Verification items for the finished model (mm, model axes). A direction names the side the tool comes from. Coordinates: 2 decimals unless noted, no trailing zeros. Write each loop counter-clockwise with the first axis right and the second up, starting at its lowest first coordinate (ties: lowest second). Pieces come first, ordered by that corner, then holes. Notation, with made-up numbers: M 47,-17 L 70,-17 A22 ccw 70,12 Z; hole C 84,26 d11. An arc over 180 degrees is marked long. Answer in a Markdown table with one row per item.
from build123d import *

# Parameters (mm, degrees)
CROQUIS1_W               = 12.68
CROQUIS1_H               = 12.6
SALIENTE_EXTRUIR1_DEPTH  = 5
SALIENTE_EXTRUIR3_DEPTH  = 5
SALIENTE_EXTRUIR4_DEPTH  = 12.5
CROQUIS2_W               = 12.6
CROQUIS2_H               = 5
CORTAR_EXTRUIR1_DEPTH    = 127.5
CROQUIS3_W               = 4.8
CROQUIS3_H               = 5
CORTAR_EXTRUIR2_DEPTH    = 255
CROQUIS4_W               = 116.76
CROQUIS4_H               = 10
CROQUIS4_H_2             = 12.5
SALIENTE_EXTRUIR5_DEPTH  = 25
CROQUIS5_R               = 4.5
CORTAR_EXTRUIR3_DEPTH    = 155
CROQUIS6_R               = 7.7
CORTAR_EXTRUIR4_DEPTH    = 20.3
CROQUIS7_R               = 7.7
SALIENTE_EXTRUIR6_DEPTH  = 5
CORTAR_EXTRUIR5_DEPTH    = 25.2
CROQUIS9_W               = 1
CROQUIS9_H               = 10
CORTAR_EXTRUIR6_DEPTH    = 4.8
CROQUIS10_W              = 117.76
CROQUIS10_H              = 0.4
CORTAR_EXTRUIR7_DEPTH    = 10
CROQUIS11_R              = 2
CORTAR_EXTRUIR8_DEPTH    = 10
CROQUIS12_W              = 3
CROQUIS12_H              = 7.5
CORTAR_EXTRUIR9_DEPTH    = 220
CORTAR_EXTRUIR10_DEPTH   = 220
SALIENTE_EXTRUIR7_DEPTH  = 16.68
CROQUIS15_R              = 7.7
SALIENTE_EXTRUIR8_DEPTH  = 1
CROQUIS16_R              = 7.7
CROQUIS16_R_2            = 4.5
SALIENTE_EXTRUIR9_DEPTH  = 1.8
SALIENTE_EXTRUIR10_DEPTH = 1
CROQUIS18_W              = 0.78
CROQUIS18_H              = 5
SALIENTE_EXTRUIR11_DEPTH = 31
SALIENTE_EXTRUIR12_DEPTH = 0.78
CORTAR_EXTRUIR11_DEPTH   = 220.78
CROQUIS21_R              = 2
CORTAR_EXTRUIR12_DEPTH   = 220.78
CROQUIS22_W              = 0.2
CROQUIS22_H              = 10
SALIENTE_EXTRUIR13_DEPTH = 30.78


with BuildPart() as part:
    # Croquis1 → Saliente-Extruir1 (new body)
    with BuildSketch(Plane(origin=(0, 0, 0), x_dir=(1, 0, 0), z_dir=(0, 1, 0))):
        with Locations((-52.04, 18.9)):
            Rectangle(CROQUIS1_W, CROQUIS1_H)
        Polygon((-45.7, 12.6), (-58.38, 12.6), (-58.38, -4.8), (58.38, -4.8), (58.38, 12.6), (45.7, 12.6), (45.7, 0), (-45.7, 0), align=None)
        with Locations((52.04, 18.9)):
            Rectangle(CROQUIS1_W, CROQUIS1_H)
    extrude(amount=SALIENTE_EXTRUIR1_DEPTH)

    # Croquis1_4 → Saliente-Extruir3 (add)
    with BuildSketch(Plane(origin=(0, 0, 0), x_dir=(1, 0, 0), z_dir=(0, 1, 0))):
        Polygon((-45.7, 12.6), (-58.38, 12.6), (-58.38, -4.8), (58.38, -4.8), (58.38, 12.6), (45.7, 12.6), (45.7, 0), (-45.7, 0), align=None)
    extrude(amount=-SALIENTE_EXTRUIR3_DEPTH)

    # Croquis1_5 → Saliente-Extruir4 (add)
    with BuildSketch(Plane(origin=(0, 0, 0), x_dir=(1, 0, 0), z_dir=(0, 1, 0))):
        Polygon((-45.7, 12.6), (-58.38, 12.6), (-58.38, -4.8), (58.38, -4.8), (58.38, 12.6), (45.7, 12.6), (45.7, 0), (-45.7, 0), align=None)
    extrude(amount=SALIENTE_EXTRUIR4_DEPTH)

    # Croquis2 → Cortar-Extruir1 (cut, symmetric)
    with BuildSketch(Plane.ZY.offset(-45.7)):
        with Locations((-6.3, -2.5)):
            Rectangle(CROQUIS2_W, CROQUIS2_H)
    extrude(amount=CORTAR_EXTRUIR1_DEPTH, both=True, mode=Mode.SUBTRACT)

    # Croquis3 → Cortar-Extruir2 (cut)
    with BuildSketch(Plane.ZY.offset(58.38)):
        with Locations((2.4, -2.5)):
            Rectangle(CROQUIS3_W, CROQUIS3_H)
    extrude(amount=-CORTAR_EXTRUIR2_DEPTH, mode=Mode.SUBTRACT)

    # Croquis4 → Saliente-Extruir5 (add)
    with BuildSketch(Plane.XY.offset(4.8)):
        with Locations((0, -5)):
            Rectangle(CROQUIS4_W, CROQUIS4_H)
        with Locations((0, 6.25)):
            Rectangle(CROQUIS4_W, CROQUIS4_H_2)
        with Locations((0, 17.5)):
            Rectangle(CROQUIS4_W, CROQUIS4_H)
    extrude(amount=SALIENTE_EXTRUIR5_DEPTH)

    # Croquis5 → Cortar-Extruir3 (cut)
    with BuildSketch(Plane.ZY.offset(58.38)):
        with Locations((20.1, 4)):
            Circle(CROQUIS5_R)
    extrude(amount=-CORTAR_EXTRUIR3_DEPTH, mode=Mode.SUBTRACT)

    # Croquis6 → Cortar-Extruir4 (cut)
    with BuildSketch(Plane.ZY.offset(58.38)):
        with Locations((20.1, 4)):
            Circle(CROQUIS6_R)
    cortar_extruir4 = extrude(amount=-CORTAR_EXTRUIR4_DEPTH, mode=Mode.SUBTRACT)

    # Simetr_a1: Cortar-Extruir4 across plane
    add(cortar_extruir4.mirror(Plane(origin=(0, 0, 0), x_dir=(0, 0, 1), z_dir=(1, 0, 0))), mode=Mode.SUBTRACT)

    # Croquis7 → Saliente-Extruir6 (add)
    with BuildSketch(Plane.ZY.offset(58.38)):
        Polygon((-25.2, 5), (-25.2, -10), (29.8, -10), (29.8, 22.5), (4.8, 22.5), (4.8, 12.5), (-12.6, 12.5), (-12.6, 5), align=None)
        with Locations((20.1, 4)):
            Circle(CROQUIS7_R, mode=Mode.SUBTRACT)
    saliente_extruir6 = extrude(amount=SALIENTE_EXTRUIR6_DEPTH)

    # Simetr_a2: Saliente-Extruir6 across plane
    add(saliente_extruir6.mirror(Plane(origin=(0, 0, 0), x_dir=(0, 0, 1), z_dir=(1, 0, 0))))

    # Croquis8 → Cortar-Extruir5 (cut)
    with BuildSketch(Plane(origin=(0, 0, -25.2), x_dir=(-1, 0, 0), z_dir=(0, 0, -1))):
        Polygon((-58.38, -10), (-59.38, -10), (-59.38, 0), (-58.38, 0), (-46.7, 0), (-46.7, 5), (-46.7, 12.5), (-42.184789705, 12.5), (-42.184789705, -10), align=None)
    extrude(amount=-CORTAR_EXTRUIR5_DEPTH, mode=Mode.SUBTRACT)

    # Croquis9 → Cortar-Extruir6 (cut)
    with BuildSketch(Plane(origin=(0, 0, 0), x_dir=(-1, 0, 0), z_dir=(0, 0, -1))):
        with Locations((-58.88, -5)):
            Rectangle(CROQUIS9_W, CROQUIS9_H)
    extrude(amount=-CORTAR_EXTRUIR6_DEPTH, mode=Mode.SUBTRACT)

    # Croquis10 → Cortar-Extruir7 (cut)
    with BuildSketch(Plane.XZ.offset(10)):
        with Locations((0.5, 5)):
            Rectangle(CROQUIS10_W, CROQUIS10_H)
    extrude(amount=-CORTAR_EXTRUIR7_DEPTH, mode=Mode.SUBTRACT)

    # Croquis11 → Cortar-Extruir8 (cut)
    with BuildSketch(Plane(origin=(0, 5, 0), x_dir=(1, 0, 0), z_dir=(0, 1, 0))):
        with Locations(Location((50.98, 15.2, 0), (0, 0, 270))):
            Circle(CROQUIS11_R)
    extrude(amount=-CORTAR_EXTRUIR8_DEPTH, mode=Mode.SUBTRACT)

    # Croquis12 → Cortar-Extruir9 (cut)
    with BuildSketch(Plane(origin=(63.38, 0, 0), x_dir=(0, 0, -1), z_dir=(1, 0, 0))):
        with Locations((11.1, 8.75)):
            Rectangle(CROQUIS12_W, CROQUIS12_H)
    extrude(amount=-CORTAR_EXTRUIR9_DEPTH, mode=Mode.SUBTRACT)

    # Croquis13 → Cortar-Extruir10 (cut)
    with BuildSketch(Plane(origin=(63.38, 0, 0), x_dir=(0, 0, -1), z_dir=(1, 0, 0))):
        Polygon((9.6, 12.5), (9.6, 5), (-4.8, 22.5), (9.6, 22.5), align=None)
    extrude(amount=-CORTAR_EXTRUIR10_DEPTH, mode=Mode.SUBTRACT)

    # Croquis14 → Saliente-Extruir7 (add)
    with BuildSketch(Plane(origin=(63.38, 0, 0), x_dir=(0, 0, -1), z_dir=(1, 0, 0))):
        Polygon((-4.8, 22.5), (3.428571429, 12.5), (-4.8, 12.5), align=None)
    saliente_extruir7 = extrude(amount=-SALIENTE_EXTRUIR7_DEPTH)

    # Simetr_a4: Saliente-Extruir7 across plane
    add(saliente_extruir7.mirror(Plane(origin=(0, 0, 0), x_dir=(0, 0, 1), z_dir=(1, 0, 0))))

    # Croquis15 → Saliente-Extruir8 (add)
    with BuildSketch(Plane(origin=(63.38, 0, 0), x_dir=(0, 0, -1), z_dir=(1, 0, 0))):
        Polygon((-29.8, 22.5), (-4.8, 22.5), (9.6, 5), (25.2, 5), (25.2, -10), (-29.8, -10), align=None)
        with Locations(Location((-20.1, 4, 0), (0, 0, 180))):
            Circle(CROQUIS15_R, mode=Mode.SUBTRACT)
    extrude(amount=SALIENTE_EXTRUIR8_DEPTH)

    # Croquis16 → Saliente-Extruir9 (add)
    with BuildSketch(Plane(origin=(38.08, 0, 0), x_dir=(0, 0, -1), z_dir=(1, 0, 0))):
        with Locations(Location((-20.1, 4, 0), (0, 0, 180))):
            Circle(CROQUIS16_R)
        with Locations(Location((-20.1, 4, 0), (0, 0, 180))):
            Circle(CROQUIS16_R_2, mode=Mode.SUBTRACT)
    extrude(amount=SALIENTE_EXTRUIR9_DEPTH)

    # Croquis17 → Saliente-Extruir10 (add)
    with BuildSketch(Plane(origin=(-46.7, 0, 0), x_dir=(0, 0, -1), z_dir=(1, 0, 0))):
        Polygon((-4.8, 12.5), (3.428571429, 12.5), (-4.8, 22.5), align=None)
    extrude(amount=SALIENTE_EXTRUIR10_DEPTH)

    # Croquis18 → Saliente-Extruir11 (add)
    with BuildSketch(Plane(origin=(0, 0, -25.2), x_dir=(-1, 0, 0), z_dir=(0, 0, -1))):
        with Locations((45.31, 2.5)):
            Rectangle(CROQUIS18_W, CROQUIS18_H)
    extrude(amount=-SALIENTE_EXTRUIR11_DEPTH)

    # Croquis19 → Saliente-Extruir12 (add)
    with BuildSketch(Plane(origin=(-45.7, 0, 0), x_dir=(0, 0, -1), z_dir=(1, 0, 0))):
        Polygon((0, 5), (9.6, 5), (-4.8, 22.5), (-4.8, 12.5), (0, 12.5), align=None)
    extrude(amount=SALIENTE_EXTRUIR12_DEPTH)

    # Croquis20 → Cortar-Extruir11 (cut)
    with BuildSketch(Plane(origin=(0, 0, -25.2), x_dir=(-1, 0, 0), z_dir=(0, 0, -1))):
        Polygon((63.38, -10), (62.58, -10), (62.58, 24.783084916), (64.574370111, 24.783084916), (64.574370111, -10), align=None)
    extrude(amount=-CORTAR_EXTRUIR11_DEPTH, mode=Mode.SUBTRACT)

    # Croquis21 → Cortar-Extruir12 (cut)
    with BuildSketch(Plane(origin=(0, 5, 0), x_dir=(1, 0, 0), z_dir=(0, 1, 0))):
        with Locations(Location((-50.22, 15.2, 0), (0, 0, 270))):
            Circle(CROQUIS21_R)
    extrude(amount=-CORTAR_EXTRUIR12_DEPTH, mode=Mode.SUBTRACT)

    # Croquis22 → Saliente-Extruir13 (add)
    with BuildSketch(Plane(origin=(0, 0, -25.2), x_dir=(-1, 0, 0), z_dir=(0, 0, -1))):
        with Locations((-59.28, -5)):
            Rectangle(CROQUIS22_W, CROQUIS22_H)
    extrude(amount=-SALIENTE_EXTRUIR13_DEPTH)


solid = part.part
1) Sectioned sample at B-B (z = -15.2). Record the cut outline in (x, y), then the cut area to 3 significant figures.
Response values:
| item | result |
|---|---|
| outline | M -62.58,-10 L -58.38,-10 L -58.38,0 L -52.22,0 L -52.22,5 L -62.58,5 Z; M -48.22,0 L -44.92,0 L -44.92,5 L -48.22,5 Z; M 46.7,0 L 48.98,0 L 48.98,5 L 46.7,5 Z; M 52.98,0 L 59.18,0 L 59.18,-10 L 64.38,-10 L 64.38,5 L 52.98,5 Z |
| area | 231 mm² |
2) Sectioned sample at A-A (x = -50.22). Record the cut outline in (y, z).
Response values:
| item | result |
|---|---|
| outline | M -10,5.2 L 0,5.2 L 0,-13.2 L 5,-13.2 L 5,-9.6 L 22.5,4.8 L 22.5,29.8 L -10,29.8 Z; M 0,-25.2 L 5,-25.2 L 5,-17.2 L 0,-17.2 Z; hole C 4,20.1 d15.4 |
3) Thickness scan on L1, parallel to X at y = 3.2, z = -15.2; L2, parallel to X at y = 1.5, z = -22; L3, parallel to Y at x = 7, z = 20. Record the ranges inside material, lowest first. Write a range as [from, to].
Response values:
| item | result |
|---|---|
| L1 | x = [-62.58, -52.22], [-48.22, -44.92], [46.7, 48.98], [52.98, 64.38] |
| L2 | x = [-62.58, -44.92], [46.7, 64.38] |
| L3 | y = [-10, -0.5], [8.5, 22.5] |
4) Release check for a two-part mould opening along Z. For faces 1 (the face through (0, 18, 4.8)), 2 (the face through (-50.158, -3.517, 18.431)), 3 (the face through (-62.58, 2, 2)) record: +Z half, -Z half, draft (parallel to the pull), parting line (faces both ways), or undercut.
Response values:
| item | result |
|---|---|
| face 1 | -Z half |
| face 2 | undercut |
| face 3 | draft |
5) Sectioned sample at D-D (z = 20.1). Record the cut outline in (x, y), then the cut area to 3 significant figures.
Response values:
| item | result |
|---|---|
| outline | M -62.58,-10 L 64.38,-10 L 64.38,-3.7 L 39.88,-3.7 L 39.88,-0.5 L -38.08,-0.5 L -38.08,-3.7 L -62.58,-3.7 Z; M -62.58,11.7 L -38.08,11.7 L -38.08,8.5 L 39.88,8.5 L 39.88,11.7 L 64.38,11.7 L 64.38,22.5 L -62.58,22.5 Z |
| area | 2,670 mm² |
6) Depth check by flat-ended pin: pin 1 (12.5 mm diameter, centred on x = -50.5, z = -13.5, fed in from +Y); pin 2 (6.5 mm diameter, centred on x = 50.98, z = -15.2, fed in from +Y); pin 3 (1.4 mm diameter, centred on x = 17, z = 3, fed in from +Y). Enter the tip coordinate at first touch or a pass-through.
Response values:
| item | result |
|---|---|
| pin 1 | stops at y = 7.86 |
| pin 2 | stops at y = 5 |
| pin 3 | stops at y = 12.5 |
7) Sectioned sample at C-C (x = 27.5). Record the cut outline in (y, z), then the cut area to 3 significant figures.
Response values:
| item | result |
|---|---|
| outline | M -10,5.2 L 0,5.2 L 0,0 L 12.5,0 L 12.5,4.8 L 22.5,4.8 L 22.5,29.8 L -10,29.8 Z; hole C 4,20.1 d9 |
| area | 805 mm² |
8) Tool access check on faces 4 (the face through (46.7, 5, -8)), 5 (the face through (0, 6, 0)), 6 (the face through (1, 0, 2)), 7 (the face through (-38.08, 0.7, 23.4)). Record the directions out of +Z, -Z, +X, -X, +Y, -Y that give a thin tool (end or side, any length) a straight path to the whole face; none if there is none.
Response values:
| item | result |
|---|---|
| face 4 | -Z, +Y |
| face 5 | -Z, +Y, -Y |
| face 6 | -Z, -Y |
| face 7 | -X |
